Build history of the part. All positions in model axes, mm. A direction names the side the tool comes from. Round coordinates to 2 decimals unless told otherwise and drop trailing zeros. Order: outer loops, then holes, each group sorted by start corner. A loop starts at its lowest first (then second) coordinate and runs counter-clockwise, first axis right, second up. Notation, with made-up numbers: M 5.5,48.5 L 26.5,48.5 A30 cw 26.5,86.5 Z; hole C 9,16 d3. An arc over 180 degrees is marked long. One line per item, written item: value. Start each with the question number.
Item 1: Probe L1, parallel to Z at x = 1, y = -2.65; L2, parallel to Z at x = 6, y = -1; L3, parallel to X at y = -1.6, z = -13.5. List the from-to ranges inside material, lowest first.
Item 2: Pin check, flat tip, straight feed: pin 1 (1.5 mm diameter, centred on y = -1.5, z = -7.5, fed in from -X). Stop position of the tip, or through.
Item 3: Tool access for faces 1 (the flat face through (10, 0, -9)), 2 (the flat face through (0, -2, -7)): list every direction of +Z, -Z, +X, -X, +Y, -Y with a clear straight run to the whole face (end or side of a thin tool).
Item 4: Band-saw the part on A-A, the plane y = -2.45. Write the cut outline in (x, z), then the cut area to 3 significant figures.
Item 5: Band-saw the part on B-B, the plane z = -8.75. Write the cut outline in (x, y), then the cut area to 3 significant figures.
Item 6: Band-saw the part on C-C, the plane x = 8. Write the cut outline in (y, z), then the cut area to 3 significant figures.
```python
from build123d import *

# Parameters (mm, degrees)
F1_DEPTH = 3.2
F2_R     = 1


with BuildPart() as f1:
    # F0 (on Front) → F1 (new body)
    with BuildSketch(Plane.XZ):
        Polygon((35, -15), (-3.2, 0), (-3.2, -5), (0, -5), (0, -10), (-3.2, -10), (-3.2, -15), (0, -15), align=None)
    extrude(amount=F1_DEPTH)

    # F2
    f2_edges = [f1.edges().sort_by_distance(p)[0] for p in [
        (35, -1.6, -15),
    ]]
    fillet(f2_edges, radius=F2_R)


solid = f1.part
```
Output:
1. L1: z = -15 to -1.65
1. L2: z = -15 to -3.61
1. L3: x = -3.2 to 30.58
2. pin 1: stops at x = 0
3. face 1: +Z, -Z, +X, -X, +Y
3. face 2: -X, +Y, -Y
4. outline: M -3.2,-15 L 29.72,-15 A1 ccw 30.08,-13.07 L -3.2,0 L -3.2,-5 L 0,-5 L 0,-10 L -3.2,-10 Z
4. area: 267 mm²
5. outline: M 0,-3.2 L 19.08,-3.2 L 19.08,0 L 0,0 Z
5. area: 61.1 mm²
6. outline: M -3.2,-15 L 0,-15 L 0,-4.4 L -3.2,-4.4 Z
6. area: 33.9 mm²
